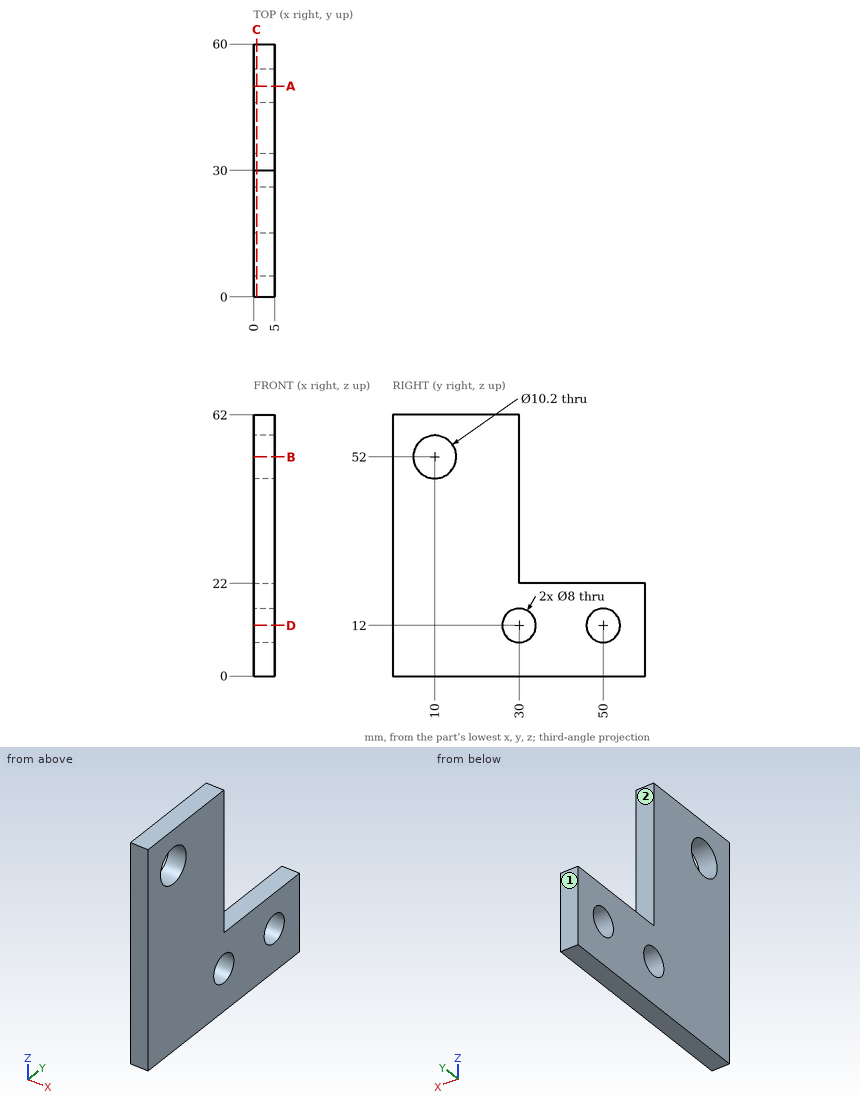
Drawing for the job (mm, zero at the part's lowest x, y, z). A direction names the side the tool comes from. Give positions to 0.01 mm unless a question says otherwise; leave off trailing zeros. Order: outer loops, then holes, each group sorted by start corner. A loop starts at its lowest first (then second) coordinate and runs counter-clockwise, first axis right, second up. Notation, with made-up numbers: M -17.75,16.5 L -9.75,16.5 A26 ccw -9.75,35.5 Z; hole C 81,17.25 d7. An arc over 180 degrees is marked long. Write item = value, one per line. Start each with the question number.
(1) Slice it at B-B on z = 52. Write the cut outline in (x, y).
(2) Probe L1, parallel to Y at x = 2.5, z = 12; L2, parallel to Y at x = 2.6, z = 52; L3, parallel to Y at x = 0.65, z = 27.5. List the from-to ranges inside material, lowest first. Write a range as [from, to].
(3) Pin check, flat tips, straight feed: pin 1 Ø2.5 at (x, z) = (2.5, 34.5) entering from +Y; pin 2 Ø2.5 at (x, y) = (3.5, 43.5) entering from +Z. Stop position of each tip, or through.
(4) Which spindle directions (+Z, -Z, +X, -X, +Y, -Y) get a long thin tool onto all of the face, cutting with end or side? Do the marked faces 1 and 2. Say none if no direction does.
(5) Slice it at C-C on x = 0.7. Write the cut outline in (y, z).
(6) Slice it at A-A on y = 50. Write the cut outline in (x, z), plus the area to 3 significant figures.
(7) Slice it at D-D on z = 12. Write the cut outline in (x, y).
Responses:
q1.outline = M 0,0 L 5,0 L 5,4.9 L 0,4.9 Z; M 0,15.1 L 5,15.1 L 5,30 L 0,30 Z
q2.L1 = [0, 26], [34, 46], [54, 60]
q2.L2 = [0, 4.9], [15.1, 30]
q2.L3 = [0, 30]
q3.pin_1 = 30
q3.pin_2 = 22
q4.face_1 = +Z, -Z, +X, -X, +Y
q4.face_2 = +Z, +X, -X, +Y
q5.outline = M 0,0 L 60,0 L 60,22 L 30,22 L 30,62 L 0,62 Z; hole C 10,52 d10.2; hole C 30,12 d8; hole C 50,12 d8
q6.outline = M 0,0 L 5,0 L 5,8 L 0,8 Z; M 0,16 L 5,16 L 5,22 L 0,22 Z
q6.area = 70.0 mm2
q7.outline = M 0,0 L 5,0 L 5,26 L 0,26 Z; M 0,34 L 5,34 L 5,46 L 0,46 Z; M 0,54 L 5,54 L 5,60 L 0,60 Z
